For this review, take the finished solid that the model builds, in its own axes (mm). Coordinates: 2 decimals unless noted, no trailing zeros. Write each loop counter-clockwise with the first axis right and the second up, starting at its lowest first coordinate (ties: lowest second). Pieces come first, ordered by that corner, then holes. Notation, with made-up numbers: (43, -0.75) -> (74, -0.75) arc R18 cw to (74, 25.25) -> close; hole circle Ø4 at (-25, 84.25). An arc over 180 degrees is marked (long way). Put each result on its own line as item: value. Start each with the question number.
Item 1: The part is to be moulded in two halves that separate along X. For faces 1 (the flat face through (0, -32, 0)), 2 (the cylindrical face through (1.987, -0.626, 1.479)), 3 (the flat face through (4, -35, 2)), say which applies: +X half, -X half, draft (parallel to the pull), parting line (faces both ways), or undercut.
Item 2: To check wall thickness, follow L1, parallel to Y at x = 0, z = 0.7; L2, parallel to X at y = 0, z = 2.15; L3, parallel to X at y = -0.5, z = 2.7. State the ranges of each line that lie inside material, in increasing order.
Item 3: Consider section A-A on x = 0. Give the boundary of the cut face in (y, z).
Item 4: Insertion check: P1, Ø3.5, axis at x = 0, y = 0, coming from the -Z side. The pin has a flat end and moves straight along its axis. Give the tip position at first contact, or say it passes through.
Item 5: Consider section B-B on z = 2.25. Give the boundary of the cut face in (x, y), and give its area (3 significant figures).
Autodesk Inventor part; units mm, degrees
ref_plane "YZ Plane" through (0, 0, 0) normal (1, 0, 0) x (0, 1, 0)
ref_plane "XZ Plane" through (0, 0, 0) normal (0, 1, 0) x (-1, 0, 0)
ref_plane "XY Plane" through (0, 0, 0) normal (0, 0, 1) x (1, 0, 0)
sketch "Sketch1" plane through (0, 0, 0) normal (0, 0, 1) x (1, 0, 0)
  circle A0 centre (0, 0) radius 2.0828
  dimension "d0" = 4.1656
sketch "Sketch2" plane through (0, 0, 0) normal (0, 0, 1) x (1, 0, 0)
  circle A0 centre (0, 0) radius 4
  dimension "d1" = 8
extrude "Extrusion1" add sketch "Sketch2" along normal blind 3
sketch "Sketch3" plane through (0, 0, 3) normal (0, 0, 1) x (1, 0, 0)
  circle A0 centre (0, 0) radius 4
  line L0 (-4, 0) -> (4, 0)
  line L1 (4, 0) -> (4, -70)
  line L2 (4, -70) -> (-4, -70)
  line L3 (-4, -70) -> (-4, 0)
  dimension "d4" = 70
extrude "Extrusion2" add sketch "Sketch3" against normal blind 3 contours L1 L2 L3 A0
extrude "Extrusion3" cut sketch "Sketch1" along normal blind 5
properties part number "Finger"
Return value:
1. face 1: draft
1. face 2: undercut
1. face 3: +X half
2. L1: -70 to -2.08, 2.08 to 4
2. L2: -4 to -2.08, 2.08 to 4
2. L3: -4 to -2.02, 2.02 to 4
3. outline: (-70, 0) -> (-2.08, 0) -> (-2.08, 3) -> (-70, 3) -> close; (2.08, 0) -> (4, 0) -> (4, 3) -> (2.08, 3) -> close
4. P1: through
5. outline: (-4, -70) -> (4, -70) -> (4, 0) arc R4 ccw to (-4, 0) -> close; hole circle Ø4.17 at (0, 0)
5. area: 572 mm^2
